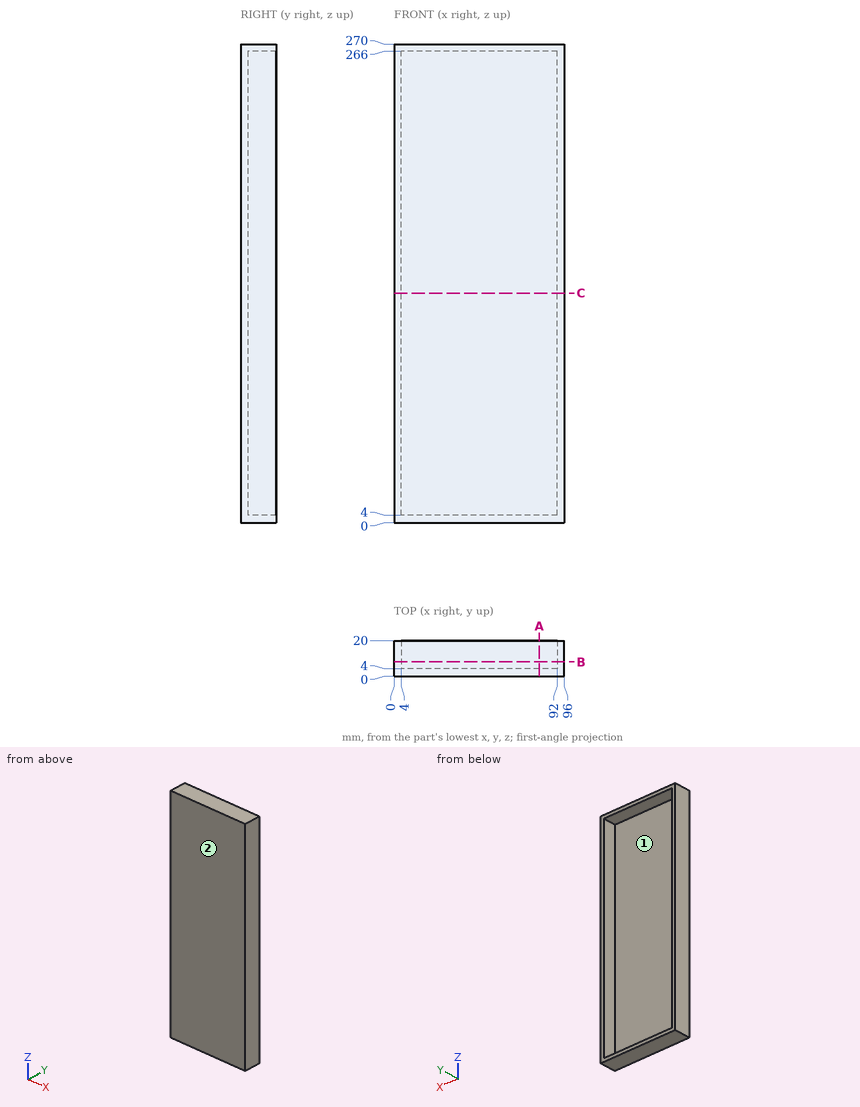
The figure shows three views and two pictorial views of one solid part (mm, origin at its lowest corner). Answer the questions. Round coordinates to 2 decimals unless told otherwise and drop trailing zeros. Loops run counter-clockwise (first coordinate to the right, second up) from the corner with the lowest first, then second, coordinate; pieces in that order, holes last. Notation, with made-up numbers: (89.5, -38.75) - (141.5, -38.75) arc R26 ccw to (141.5, -10.75) - close; hole circle Ø5 at (78.25, -29.5). An arc over 180 degrees is marked (long way). Use one line per item in the form item = value. Start each with the question number.
(1) Find section C-C on z = 129.5. Determine the outline of the cut face in (x, y), and give its area (3 significant figures).
(2) Determine the mould class of the marked faces 1 and 2 for opening direction X: +X half, -X half, draft (parallel to the pull), parting line (faces both ways), or undercut.
(3) Find section A-A on x = 82. Determine the outline of the cut face in (y, z), and give its area (3 significant figures).
(4) Find section B-B on y = 8. Determine the outline of the cut face in (x, z).
(5) Consider line 1 (X direction, y = 6.75, z = 227); line 2 (Z direction, x = 30.5, y = 18.25); line 3 (Y direction, x = 69, z = 117.5). Determine where each line is inside the solid, lowest interval first.
(6) Flat-ended cylindrical pins translate along their axes: P1, Ø8, axis at y = 14.5, z = 107.5, coming from the -X side; P2, Ø4, axis at x = 35, z = 218, coming from the +Y side. Find the tip coordinate at first contact, or state that the pin passes through.
Answer list:
q1.outline = (0, 0) - (96, 0) - (96, 20) - (92, 20) - (92, 4) - (4, 4) - (4, 20) - (0, 20) - close
q1.area = 512 mm^2
q2.face_1 = undercut
q2.face_2 = draft
q3.outline = (0, 0) - (20, 0) - (20, 4) - (4, 4) - (4, 266) - (20, 266) - (20, 270) - (0, 270) - close
q3.area = 1,210 mm^2
q4.outline = (0, 0) - (96, 0) - (96, 270) - (0, 270) - close; hole (4, 4) - (92, 4) - (92, 266) - (4, 266) - close
q5.line_1 = 0 to 4, 92 to 96
q5.line_2 = 0 to 4, 266 to 270
q5.line_3 = 0 to 4
q6.P1 = 0
q6.P2 = 4
